Check sheet for the modelled part. Datum: model origin and axes. Units: mm. A direction names the side the tool comes from. Coordinates: 2 decimals unless noted, no trailing zeros. Loops run counter-clockwise (first coordinate to the right, second up) from the corner with the lowest first, then second, coordinate; pieces in that order, holes last. Notation, with made-up numbers: (-24.5, 15) -> (13.5, 15) arc R26 cw to (13.5, 44) -> close; hole circle Ø1 at (59, 63.25). An arc over 180 degrees is marked (long way). Use CSV: the item, a comma, the result in double quotes. Start each with the question number.
1. Sectioned sample at A-A, the plane y = 37. Record the cut outline in (x, z).
2. Set-up check for faces 1 (the face through (-0.238, -33.065, -14.096)), 2 (the face through (-20, 27, -3)): record each of +Z, -Z, +X, -X, +Y, -Y from which the full face is reachable in a straight line by a thin tool's end or side.
3. Thickness scan on L1, parallel to Z at x = -13, y = 36.5; L2, parallel to X at y = -10.5, z = -6. Record the ranges inside material, lowest first.
4. Gauge pin test, flat ends, axial feed: pin 1 (3 mm diameter, centred on x = -10.5, y = -31.5, fed in from +Z); pin 2 (7 mm diameter, centred on x = -1, z = 5.5, fed in from +Y). Record the tip position at first contact, or that the pin passes through.
5. Release check for a two-part mould opening along Z. For faces 3 (the face through (-15.545, -33.827, 15.622)), 4 (the face through (-10.1, -66.8, 4.3)), 5 (the face through (0, -65.344, -1)), 6 (the face through (0, -68.344, -2)) record: pulls with the +Z half, pulls with the -Z half, needs draft (parallel to the pull), parting line crosses it, or undercut.
```python
from build123d import *

# Parameters (mm, degrees)
F0_W          = 40
F0_H          = 40
F1_DEPTH      = 68.34402
F1_TAPER      = 5
F1_DEPTH_BACK = 54.92041
F2_T1_DEPTH   = 129.92041
F2_T3_DEPTH   = 143.2975946274
F2_T5_DEPTH   = 143.2975946274
F3_T          = 3
F5_D          = 5


# Not quite as in the source:
# - a fillet or chamfer that OpenCascade refuses, or shapes differently, is made with other operations: its cross-section is extruded or revolved along the edge and cut away or added
# - a shell that OpenCascade refuses in one call is made with other operations: the cavity is built on its own and cut out


with BuildPart() as f1:
    # F0 (on Front) → F1 (new body, two sides)
    with BuildSketch(Plane.XZ) as f1_sk:
        Rectangle(F0_W, F0_H)
    extrude(amount=F1_DEPTH, taper=F1_TAPER)
    extrude(f1_sk.sketch, amount=-F1_DEPTH_BACK)

    # F2: fillet of radius 5 on 4 edges, made by hand

    # F2_s2 → F2_t1 (cut)
    with BuildSketch(Plane.XZ.offset(-67.42041)):
        with BuildLine():
            ThreePointArc((20, 15), (18.5355339059, 18.5355339059), (15, 20))
            Line((15, 20), (20, 20))
            Line((20, 20), (20, 15))
        make_face()
        with BuildLine():
            ThreePointArc((-15, 20), (-18.5355339059, 18.5355339059), (-20, 15))
            Line((-20, 15), (-20, 20))
            Line((-20, 20), (-15, 20))
        make_face()
    extrude(amount=F2_T1_DEPTH, mode=Mode.SUBTRACT)

    # F2_s4 → F2_t3 (cut)
    with BuildSketch(Plane(origin=(5.6871501966, 65.0044242011, 5.6871501966), x_dir=(0.9961946981, -0.0871557427, 0), z_dir=(-0.0868265939, -0.9924325091, -0.0868265939))):
        with BuildLine():
            ThreePointArc((19.9238939618, 14.8109575307), (18.4728306397, 18.3330376627), (14.9618745793, 19.8108132759))
            Line((14.9618745793, 19.8108132759), (19.9238939618, 19.7731200764))
            Line((19.9238939618, 19.7731200764), (19.9238939618, 14.8109575307))
        make_face()
    extrude(amount=F2_T3_DEPTH, mode=Mode.SUBTRACT)

    # F2_s6 → F2_t5 (cut)
    with BuildSketch(Plane(origin=(-5.6871501966, 65.0044242011, 5.6871501966), x_dir=(0.9961946981, 0.0871557427, 0), z_dir=(0.0868265939, -0.9924325091, -0.0868265939))):
        with BuildLine():
            ThreePointArc((-14.9618745793, 19.8108132759), (-18.4728306397, 18.3330376627), (-19.9238939618, 14.8109575307))
            Line((-19.9238939618, 14.8109575307), (-19.9238939618, 19.7731200764))
            Line((-19.9238939618, 19.7731200764), (-14.9618745793, 19.8108132759))
        make_face()
    extrude(amount=F2_T5_DEPTH, mode=Mode.SUBTRACT)

    # F3: shell of thickness 3, made by hand


with BuildPart() as f3_core1:
    # F3_t2: copy of F1
    add(f1.part)

    # the walls: a layer under each face that stays
    f3_faces = [f3_core1.faces().sort_by_distance(p)[0] for p in [
        (20, 27.460205, -2.5),
        (17.0103365151, -34.17201, -2.1182047008),
        (18.5355339059, 27.415284207, 18.5355339059),
        (0, 27.460205, -20),
        (0, -34.17201, -17.0103365151),
        (0, -68.34402, -1.4566061483),
        (15.5420062021, -34.3060178162, 15.5420062021),
        (0, 27.460205, 20),
        (0, -34.17201, 17.0103365151),
        (-20, 27.460205, -2.5),
        (-18.5355339059, 27.415284207, 18.5355339059),
        (-17.0103365151, -34.17201, -2.1182047008),
        (-15.5420062021, -34.3060178161, 15.5420062021),
    ]]
    thicken(f3_faces, amount=-F3_T, mode=Mode.SUBTRACT)


with BuildPart() as f1_1:
    add(f1.part)

    # what is left inside the walls is the cavity
    f3_cavity = [f3_core1.part.solids().sort_by_distance(p)[0] for p in [
        (0, 36.657268, -16.97),
    ]]
    add(f3_cavity, mode=Mode.SUBTRACT)

    # F5 (through all)
    with Locations(Plane.XZ.offset(68.34402)):
        with Locations((-5, -9), (-7.7271993353, 3.5151276782)):
            Hole(F5_D / 2)


solid = f1_1.part
```
Completed:
1,outline,"(-20, -20) -> (20, -20) -> (20, 15) arc R5 ccw to (15, 20) -> (-15, 20) arc R5 ccw to (-20, 15) -> close; hole (-17, -17) -> (17, -17) -> (17, 15) arc R2 ccw to (15, 17) -> (-15, 17) arc R2 ccw to (-17, 15) -> close"
2,face 1,"+Y"
2,face 2,"+Z, -Z, -X, +Y, -Y"
3,L1,"-20 to -17, 17 to 20"
3,L2,"-19.08 to -16.07, 16.07 to 19.08"
4,pin 1,"z = 17.38"
4,pin 2,"y = -65.34"
5,face 3,"pulls with the +Z half"
5,face 4,"undercut"
5,face 5,"undercut"
5,face 6,"needs draft"
